Autodesk Inventor part; units mm, degrees
ref_plane "YZ Plane" through (0, 0, 0) normal (1, 0, 0) x (0, 1, 0)
ref_plane "XZ Plane" through (0, 0, 0) normal (0, 1, 0) x (-1, 0, 0)
ref_plane "XY Plane" through (0, 0, 0) normal (0, 0, 1) x (1, 0, 0)
sketch "Sketch1" plane through (0, 0, 0) normal (0, 0, 1) x (1, 0, 0)
  circle A0 centre (0, 0) radius 20.5
  circle A1 centre (0, 0) radius 17.5
  line L0 (-1.9, 17.5) -> (1.9, 17.5)
  line L1 (-1.9, 17.5) -> (-1.9, 22.5)
  line L2 (-1.9, 22.5) -> (1.9, 22.5)
  line L3 (1.9, 22.5) -> (1.9, 17.5)
  circle A2 centre (0, 22.5) radius 1.9
  circle A3 centre (-17.5912, 14.0285) radius 1.9
  line L4 (-16.4066, 15.514) -> (-12.4974, 12.3966)
  line L5 (-18.7758, 12.543) -> (-16.4066, 15.514)
  line L6 (-14.8667, 9.4256) -> (-18.7758, 12.543)
  line L7 (-14.8667, 9.4256) -> (-12.4974, 12.3966)
  circle A4 centre (-21.9359, -5.0067) radius 1.9
  line L8 (-22.3587, -3.1544) -> (-17.484, -2.0418)
  line L9 (-21.5131, -6.8591) -> (-22.3587, -3.1544)
  line L10 (-16.6384, -5.7465) -> (-21.5131, -6.8591)
  line L11 (-16.6384, -5.7465) -> (-17.484, -2.0418)
  circle A5 centre (-9.7624, -20.2718) radius 1.9
  line L12 (-11.4742, -19.4474) -> (-9.3048, -14.9426)
  line L13 (-8.0505, -21.0962) -> (-11.4742, -19.4474)
  line L14 (-5.8811, -16.5913) -> (-8.0505, -21.0962)
  line L15 (-5.8811, -16.5913) -> (-9.3048, -14.9426)
  circle A6 centre (9.7624, -20.2718) radius 1.9
  line L16 (8.0505, -21.0962) -> (5.8811, -16.5913)
  line L17 (11.4742, -19.4474) -> (8.0505, -21.0962)
  line L18 (9.3048, -14.9426) -> (11.4742, -19.4474)
  line L19 (9.3048, -14.9426) -> (5.8811, -16.5913)
  circle A7 centre (21.9359, -5.0067) radius 1.9
  line L20 (21.5131, -6.8591) -> (16.6384, -5.7465)
  line L21 (22.3587, -3.1544) -> (21.5131, -6.8591)
  line L22 (17.484, -2.0418) -> (22.3587, -3.1544)
  line L23 (17.484, -2.0418) -> (16.6384, -5.7465)
  circle A8 centre (17.5912, 14.0285) radius 1.9
  line L24 (18.7758, 12.543) -> (14.8667, 9.4256)
  line L25 (16.4066, 15.514) -> (18.7758, 12.543)
  line L26 (12.4974, 12.3966) -> (16.4066, 15.514)
  line L27 (12.4974, 12.3966) -> (14.8667, 9.4256)
  line L28 (-1.9, 17.5) -> (5.1, 17.5)
  line L29 (5.1, 17.5) -> (5.1, 0)
  line L30 (5.1, 0) -> (-1.9, 0)
  line L31 (-1.9, 0) -> (-1.9, 17.5)
  line L32 (-0.5871, -1.807) -> (-17.2306, 3.6008)
  line L33 (-17.2306, 3.6008) -> (-15.0675, 10.2582)
  line L34 (-15.0675, 10.2582) -> (1.576, 4.8504)
  line L35 (1.576, 4.8504) -> (-0.5871, -1.807)
  line L36 (1.5371, -1.1168) -> (-8.7491, -15.2746)
  line L37 (-8.7491, -15.2746) -> (-14.4122, -11.1601)
  line L38 (-14.4122, -11.1601) -> (-4.126, 2.9977)
  line L39 (-4.126, 2.9977) -> (1.5371, -1.1168)
  line L40 (1.5371, 1.1168) -> (11.8234, -13.041)
  line L41 (11.8234, -13.041) -> (6.1603, -17.1555)
  line L42 (6.1603, -17.1555) -> (-4.126, -2.9977)
  line L43 (-4.126, -2.9977) -> (1.5371, 1.1168)
  line L44 (-0.5871, 1.807) -> (16.0564, 7.2148)
  line L45 (16.0564, 7.2148) -> (18.2195, 0.5574)
  line L46 (18.2195, 0.5574) -> (1.576, -4.8504)
  line L47 (1.576, -4.8504) -> (-0.5871, 1.807)
  point P0 (-17.1432, 11.241)
  point P1 (-20.3228, -2.6897)
  point P2 (-21.5131, -6.8591)
  point P3 (-19.4772, -6.3944)
  point P4 (-10.5682, -17.566)
  point P5 (-7.1445, -19.2147)
  point P6 (7.1445, -19.2147)
  point P7 (10.5682, -17.566)
  point P8 (19.4772, -6.3944)
  point P9 (22.3587, -3.1544)
  point P10 (20.3228, -2.6897)
  point P11 (17.1432, 11.241)
  point P12 (16.4066, 15.514)
  point P13 (14.7739, 14.212)
  point P14 (1.9, 20.4118)
  point P15 (-1.9, 20.4118)
  point P16 (-14.7739, 14.212)
  point P17 (-17.1322, 3.5688)
  point P18 (-6.2743, 0.0409)
  point P19 (-13.9657, -10.5455)
  point P20 (11.7626, -12.9573)
  point P21 (5.052, -3.721)
  point P22 (17.497, 0.3227)
  point P23 (15.958, 7.1828)
  point P24 (5.1, 3.6549)
  point P25 (5.1, 16.7404)
  point P26 (-8.6883, -15.1909)
  point P27 (-1.9777, -5.9546)
  point P28 (5.7138, -16.5409)
  point P29 (-1.9, 17.3966)
  point P30 (-1.9, 5.9798)
  point P31 (-14.3451, 10.0234)
  point P32 (16.4066, 15.514)
  point P33 (22.3587, -3.1544)
  point P34 (11.4742, -19.4474)
  point P35 (-21.5131, -6.8591)
  dimension "d0" = 35
  dimension "d1" = 41
  dimension "d2" = 3.8
  dimension "d4" = 1.9
  dimension "d5" = 17.5
  dimension "d6" = 5
  dimension "d7" = 3.8
  dimension "d11" = 360
  dimension "d13" = 7
  dimension "d14" = 17.5
  dimension "d17" = 360
extrude "Extrusion1" add sketch "Sketch1" along normal mid plane 12 contours A0 L22 L23 A1 L46 L45 L44 L27 L24 | L24 L27 L26 A0 | A0 L20 L23 L22 | L26 L27 A1 L29 L28 L3 A0 | A0 L18 L19 L41 L40 A1 L23 L20 | L3 L0 L1 A0 | A0 L16 L42 L41 L19 L18 | L1 L31 A1 L7 L4 A0 | L28 L29 A1 L0 | L44 L45 A1 | A1 L46 L40 L30 L29 L44 | L29 L44 L35 L34 L31 A1 | A0 L14 L15 A1 L42 L16 | L40 L41 A1 | A1 L42 L36 L47 L46 L40 | L4 L7 L34 L33 L6 A0 | L0 A1 L31 | L45 L46 A1 | L29 L30 L40 L43 L35 L44 | A0 L12 L15 L37 L36 L14 | L42 A1 L19 L16 | L16 L19 L41 L42 | L19 A1 L41 | L46 L47 L36 L39 L30 L40 | L6 L33 L32 A1 L11 L8 A0 | L44 L47 L39 L31 L34 L35 | L35 L47 L44 | A0 L10 L11 A1 L38 L37 L15 L12 | L30 L43 L40 | L8 L11 L10 A0 | L33 L34 L7 L6 | L6 L7 L34 A1 L33 | A1 L34 L7 | L31 L39 L38 L32 A1 L34 | L43 L32 L38 L39 L31 L30 | L47 L36 L42 L43 L32 L35 | L30 L31 L39 | L35 L32 L43 | L39 L36 L47 | L15 L36 A1 | L36 A1 L38 L32 L43 L42 | A1 L32 L33 | L37 A1 L36 L15 | L15 L36 L37 | L37 L38 A1
extrude "Extrusion2" add sketch "Sketch1" along normal mid plane 3.7 contours A0 L22 L23 A1 L46 L45 L44 L27 L24 | L24 L27 L26 A0 | A0 L26 A8 L24 | L22 A7 L20 A0 | A0 L20 L23 L22 | L26 L27 A1 L29 L28 L3 A0 | L25 A8 | A8 L25 | A0 L18 L19 L41 L40 A1 L23 L20 | L21 A7 | A7 L21 | L3 L0 L1 A0 | A0 L1 A2 L3 | L18 A6 L16 A0 | A0 L16 L42 L41 L19 L18 | L1 L31 A1 L7 L4 A0 | A2 L2 | L2 A2 | L28 L29 A1 L0 | L44 L45 A1 | A1 L46 L40 L30 L29 L44 | L29 L44 L35 L34 L31 A1 | A0 L14 L15 A1 L42 L16 | L17 A6 | A6 L17 | L40 L41 A1 | A1 L42 L36 L47 L46 L40 | L4 L7 L34 L33 L6 A0 | A0 L6 A3 L4 | L0 A1 L31 | L45 L46 A1 | L29 L30 L40 L43 L35 L44 | L14 A5 L12 A0 | A0 L12 L15 L37 L36 L14 | L42 A1 L19 L16 | L16 L19 L41 L42 | L19 A1 L41 | L46 L47 L36 L39 L30 L40 | L6 L33 L32 A1 L11 L8 A0 | L5 A3 | A3 L5 | L44 L47 L39 L31 L34 L35 | L35 L47 L44 | A0 L10 L11 A1 L38 L37 L15 L12 | L13 A5 | A5 L13 | L30 L43 L40 | L8 L11 L10 A0 | A0 L10 A4 L8 | L33 L34 L7 L6 | L6 L7 L34 A1 L33 | A1 L34 L7 | L31 L39 L38 L32 A1 L34 | L43 L32 L38 L39 L31 L30 | L47 L36 L42 L43 L32 L35 | L30 L31 L39 | L35 L32 L43 | L39 L36 L47 | L15 L36 A1 | L36 A1 L38 L32 L43 L42 | L9 A4 | A4 L9 | A1 L32 L33 | L37 A1 L36 L15 | L15 L36 L37 | L37 L38 A1
sketch "Sketch2" plane through (0, 0, -6) normal (0, 0, -1) x (-1, 0, 0)
  circle A0 centre (0, 0) radius 1.6
  circle A1 centre (0, 0) radius 5.5
  circle A2 centre (0, 0) radius 4.1
  dimension "d23" = 3.2
  dimension "d24" = 11
  dimension "d59" = 8.2
extrude "Extrusion3" add sketch "Sketch2" along normal blind 1 contours A0 | A1 | A2
chamfer "Chamfer1" distance 1 angle 45 10 edges at (11.2745, -1.6992, 6) (10.529, 5.4189, 6) (5.1, 10.1976, 6) (-1.9, 11.6882, 6) (-8.1225, 8.0016, 6) (-11.7033, 1.8048, 6) (-10.12, -5.2523, 6) (-5.333, -10.5727, 6) (1.868, -11.2478, 6) (8.4073, -8.3391, 6)
sketch "Sketch4" plane through (0, 0, 6) normal (0, 0, 1) x (1, 0, 0)
  circle A0 centre (0, 0) radius 1.6
  dimension "d60" = 3.2
extrude "Extrusion8" cut sketch "Sketch2" along normal blind 10 and the other way blind 11 contours A2
extrude "Extrusion9" cut sketch "Sketch4" against normal up to surface (13 mm away)
fillet "Fillet2" radius 0.5 1 edges at (4.1, 0, -7)
properties part number "wheel_big"
Geometry: final body of the model. Coordinates: model frame, mm. A direction names the side the tool comes from. Coordinates: 2 decimals unless noted, no trailing zeros. Order: outer loops, then holes, each group sorted by start corner. A loop starts at its lowest first (then second) coordinate and runs counter-clockwise, first axis right, second up. Notation, with made-up numbers: (30, 57) - (79, 57) arc R31 cw to (79, 89) - close; hole circle Ø7 at (75.5, 22). An arc over 180 degrees is marked (long way). Use one line per item in the form item = value.
1) Pin query (flat end, axial travel): pin 1 (2.5 mm diameter, centred on x = -2, y = 0, fed in from -Z); pin 2 (3 mm diameter, centred on x = 0, y = 0, fed in from +Z) (3 decimals); pin 3 (2.5 mm diameter, centred on x = 10, y = -20, fed in from +Z); pin 4 (2 mm diameter, centred on y = -9, z = 2.5, fed in from +X). Return the tip coordinate at first contact, or that it passes through.
Solutions:
pin_1 = 5
pin_2 = through
pin_3 = 1.85
pin_4 = 18.87
2) Section D-D (y = 8). Return loops of the section in (x, z), then the cut area to 3 significant figures.
Solutions:
outline = (-18.87, -6) - (-8.12, -6) - (-8.12, 5) - (-11.35, 6) - (-18.87, 6) - close; (-1.9, -6) - (5.1, -6) - (5.1, 5) - (4.1, 6) - (-0.9, 6) - (-1.9, 5) - close; (15.56, -6) - (18.87, -6) - (18.87, 6) - (15.56, 6) - close
area = 250 mm^2
3) Ray query, L1, parallel to Y at x = 0, z = 2.5; L2, parallel to Y at x = 0, z = 0; L3, parallel to Y at x = -7, z = -5.25. Return the intervals inside material, ascending.
Solutions:
L1 = -20.5 to -17.5, -8.68 to -4.1, 4.1 to 20.5
L2 = -20.5 to -17.5, -8.68 to -4.1, 4.1 to 24.4
L3 = -19.27 to -16.04, -12.87 to -0.96, 0.28 to 7.64, 16.04 to 19.27
4) Section A-A (y = -7.5). Return loops of the section in (x, z).
Solutions:
outline = (-19.08, -6) - (-15.81, -6) - (-15.81, 6) - (-19.08, 6) - close; (-11.75, -6) - (-3.1, -6) - (-3.1, 5) - (-4.34, 6) - (-10.52, 6) - (-11.75, 5) - close; (-0.85, -6) - (7.8, -6) - (7.8, 5) - (6.56, 6) - (0.38, 6) - (-0.85, 5) - close; (15.81, -6) - (19.08, -6) - (19.08, 6) - (15.81, 6) - close
5) Set-up query: faces 4 (the face through (2.003, -10.595, 5.493)), 5 (the face through (-1.9, 21, 0)), 6 (the face through (-15.6, 14.87, -0.03)), 7 (the face through (18, 14, 1.85)), 8 (the face through (-1.9, 12, -1)). Return all of +Z, -Z, +X, -X, +Y, -Y with unobstructed straight access to the full face (end or side cutting, diameter ignored); none if empty.
Solutions:
face_4 = +Z
face_5 = +Z, -Z, -X, +Y
face_6 = +Z, -Z, +Y
face_7 = +Z, +X, +Y
face_8 = +Z, -Z
6) Section B-B (x = 0). Return loops of the section in (y, z), then the cut area to 3 significant figures.
Solutions:
outline = (-20.5, -6) - (-17.5, -6) - (-17.5, 6) - (-20.5, 6) - close; (-8.68, -6) - (-5.5, -6) - (-5.5, -7) - (-4.6, -7) arc R0.5 ccw to (-4.1, -6.5) - (-4.1, 5) - (-1.6, 5) - (-1.6, 6) - (-6.98, 6) - (-8.68, 5) - close; (1.6, 5) - (4.1, 5) - (4.1, -6.5) arc R0.5 ccw to (4.6, -7) - (5.5, -7) - (5.5, -6) - (20.5, -6) - (20.5, -1.85) - (24.4, -1.85) - (24.4, 1.85) - (20.5, 1.85) - (20.5, 6) - (1.6, 6) - close
area = 309 mm^2
7) Mould query, pull axis X, two halves, no side actions, for faces 1 (the face through (-3, -4, -7)), 2 (the face through (-11.028, -18.52, -0.026)), 3 (the face through (-10.55, -22, -0.03)). Classes: +X half, -X half, draft (parallel to the pull), parting line (faces both ways), or undercut.
Solutions:
face_1 = draft
face_2 = -X half
face_3 = undercut
8) Section C-C (z = -3). Return loops of the section in (x, y).
Solutions:
outline = circle Ø41 at (0, 0); hole (-17.13, 3.57) arc R17.5 ccw to (-13.97, -10.55) - (-6.27, 0.04) - close; hole (-14.35, 10.02) - (-1.9, 5.98) - (-1.9, 17.4) arc R17.5 ccw to start; hole (-8.69, -15.19) arc R17.5 ccw to (5.71, -16.54) - (-1.98, -5.95) - close; hole circle Ø8.2 at (0, 0); hole (5.05, -3.72) - (11.76, -12.96) arc R17.5 ccw to (17.5, 0.32) - close; hole (5.1, 3.65) - (15.96, 7.18) arc R17.5 ccw to (5.1, 16.74) - close
